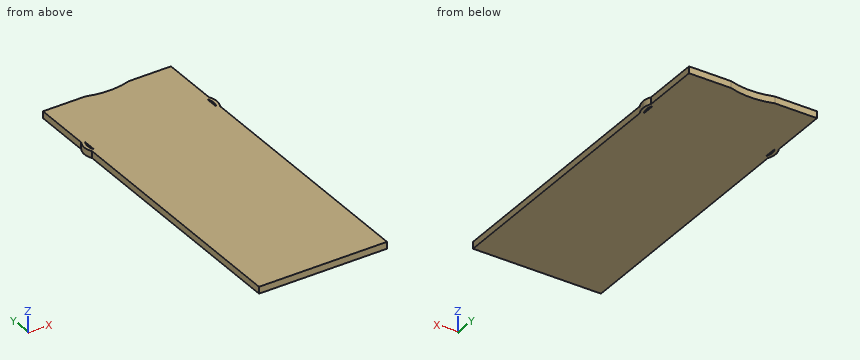
from build123d import *

# Parameters (mm, degrees)
F0_W     = 37.6
F0_H     = 96.5
F1_DEPTH = 2
F3_DEPTH = 2
F5_DEPTH = 2.001


with BuildPart() as f1:
    # F0 (on Top) → F1 (new body)
    with BuildSketch(Plane.XY):
        Rectangle(F0_W, F0_H)
    extrude(amount=F1_DEPTH)

    # F2 (on face) → F3 (join, through all)
    with BuildSketch(Plane.XY.offset(2)):
        with BuildLine():
            Line((-18.8, 26.297960033), (-18.8, 31.202039967))
            ThreePointArc((-18.8, 31.202039967), (-19.45, 28.75), (-18.8, 26.297960033))
        make_face()
        with BuildLine():
            ThreePointArc((19.45, 28.75), (19.2847413723, 30.0183650894), (18.8, 31.202039967))
            Line((18.8, 31.202039967), (18.8, 26.297960033))
            ThreePointArc((18.8, 26.297960033), (19.2847413723, 27.4816349106), (19.45, 28.75))
        make_face()
    extrude(amount=-F3_DEPTH)

    # F4 (on face) → F5 (cut, through all)
    with BuildSketch(Plane.XY.offset(2)):
        with BuildLine():
            Line((-17.9313131313, 26.7933216425), (-17.9313131313, 30.7066783575))
            ThreePointArc((-17.9313131313, 30.7066783575), (-18.45, 28.75), (-17.9313131313, 26.7933216425))
        make_face()
        with BuildLine():
            Line((17.9313131313, 30.7066783575), (17.9313131313, 26.7933216425))
            ThreePointArc((17.9313131313, 26.7933216425), (18.45, 28.75), (17.9313131313, 30.7066783575))
        make_face()
        with BuildLine():
            Line((6.4031242374, 48.25), (-6.4031242374, 48.25))
            ThreePointArc((-6.4031242374, 48.25), (0, 47.25), (6.4031242374, 48.25))
        make_face()
    extrude(amount=-F5_DEPTH, mode=Mode.SUBTRACT)


solid = f1.part
Model file for the job. Use its own axes, mm. Give positions to 0.01 mm unless a question says otherwise; leave off trailing zeros. Order: outer loops, then holes, each group sorted by start corner. A loop starts at its lowest first (then second) coordinate and runs counter-clockwise, first axis right, second up. Notation, with made-up numbers: M 40,5.25 L 64,5.25 A19 ccw 64,26.25 Z; hole C 67.5,13.5 d8. An arc over 180 degrees is marked long. Write item = value, one per line.
Q1. Flat gauge pins, fed straight in: pin 1 (0.6 mm diameter, centred on y = 29.5, z = 0.5, fed in from -X); pin 2 (0.6 mm diameter, centred on y = -14, z = 1, fed in from -X); pin 3 (1 mm diameter, centred on y = -7.5, z = 0.5, fed in from +X). Where does each tip first touch, or does it go through?
Derived:
pin_1 = -19.43
pin_2 = -18.8
pin_3 = 18.8
Q2. Cut at A-A, the plane z = 1.55. List the corners of the cut face in (x, y), then the cut area to 3 significant figures.
Derived:
outline = M -18.8,-48.25 L 18.8,-48.25 L 18.8,26.3 A4.95 ccw 18.8,31.2 L 18.8,48.25 L 6.4,48.25 A21 cw -6.4,48.25 L -18.8,48.25 L -18.8,31.2 A4.95 ccw -18.8,26.3 Z; hole M -17.93,26.79 L -17.93,30.71 A3.95 ccw Z; hole M 17.93,26.79 A3.95 ccw 17.93,30.71 Z
area = 3,620 mm2
Q3. Cut at B-B, the plane y = 36. List the corners of the cut face in (x, z).
Derived:
outline = M -18.8,0 L 18.8,0 L 18.8,2 L -18.8,2 Z
Q4. Drill centre lines: line 1 (X direction, y = 1, z = 1.5); line 2 (Y direction, x = 0.5, z = 0.75); line 3 (Y direction, x = -6, z = 1.4). Where is each one in solid material? Low to high. Write a range as [from, to].
Derived:
line_1 = [-18.8, 18.8]
line_2 = [-48.25, 47.26]
line_3 = [-48.25, 48.13]
